Read the model definition and answer for the solid it produces. Units are mm, in the model's axes. Coordinates: 2 decimals unless noted, no trailing zeros. Loops run counter-clockwise (first coordinate to the right, second up) from the corner with the lowest first, then second, coordinate; pieces in that order, holes last.
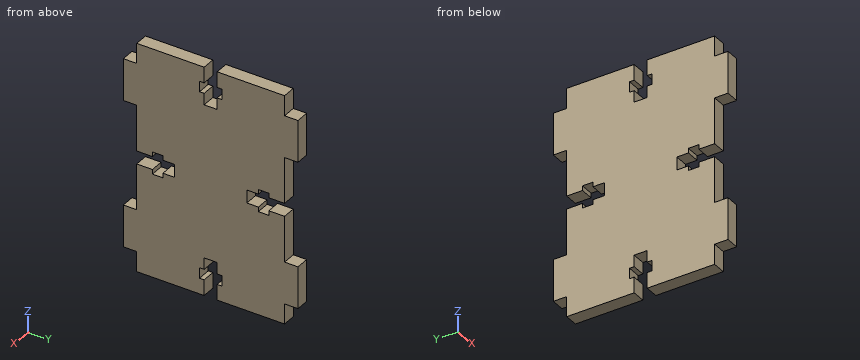
from build123d import *

# Parameters (mm, degrees)
F1_W     = 35.28
F1_H     = 54.6
F2_DEPTH = 3.2
F3_W     = 3.2
F3_H     = 10
F4_DEPTH = 3.2
F5_W     = 3.1
F5_H     = 3.75
F5_H_2   = 2.5
F5_W_2   = 1.1
F5_H_3   = 2.75
F5_W_3   = 3.75
F5_H_4   = 3.1
F5_W_4   = 2.5
F5_H_5   = 1.1
F5_W_5   = 2.75
F6_DEPTH = 3.201


with BuildPart() as f2:
    # F1 (on Right) → F2 (new body)
    with BuildSketch(Plane.YZ):
        with Locations((0, 27.3)):
            Rectangle(F1_W, F1_H)
    extrude(amount=F2_DEPTH)

    # F3 (on face) → F4 (join, through all)
    with BuildSketch(Plane.YZ.offset(3.2)):
        with Locations((-19.24, 44.8)):
            Rectangle(F3_W, F3_H)
        with Locations((-19.24, 9.8)):
            Rectangle(F3_W, F3_H)
        with Locations((19.24, 9.8)):
            Rectangle(F3_W, F3_H)
        with Locations((19.24, 44.8)):
            Rectangle(F3_W, F3_H)
    extrude(amount=-F4_DEPTH)

    # F5 (on face) → F6 (cut, through all)
    with BuildSketch(Plane.YZ.offset(3.2)):
        with Locations((0, 1.875)):
            Rectangle(F5_W, F5_H)
        with Locations((0, 5)):
            Rectangle(F5_W, F5_H_2)
        with Locations((2.1, 5)):
            Rectangle(F5_W_2, F5_H_2)
        with Locations((0, 7.625)):
            Rectangle(F5_W, F5_H_3)
        with Locations((-2.1, 5)):
            Rectangle(F5_W_2, F5_H_2)
        with Locations((-15.765, 27.3)):
            Rectangle(F5_W_3, F5_H_4)
        with Locations((-12.64, 27.3)):
            Rectangle(F5_W_4, F5_H_4)
        with Locations((-12.64, 25.2)):
            Rectangle(F5_W_4, F5_H_5)
        with Locations((-10.015, 27.3)):
            Rectangle(F5_W_5, F5_H_4)
        with Locations((-12.64, 29.4)):
            Rectangle(F5_W_4, F5_H_5)
        with Locations((12.64, 29.4)):
            Rectangle(F5_W_4, F5_H_5)
        with Locations((12.64, 27.3)):
            Rectangle(F5_W_4, F5_H_4)
        with Locations((10.015, 27.3)):
            Rectangle(F5_W_5, F5_H_4)
        with Locations((15.765, 27.3)):
            Rectangle(F5_W_3, F5_H_4)
        with Locations((12.64, 25.2)):
            Rectangle(F5_W_4, F5_H_5)
        with Locations((2.1, 49.6)):
            Rectangle(F5_W_2, F5_H_2)
        with Locations((0, 46.975)):
            Rectangle(F5_W, F5_H_3)
        with Locations((0, 49.6)):
            Rectangle(F5_W, F5_H_2)
        with Locations((0, 52.725)):
            Rectangle(F5_W, F5_H)
        with Locations((-2.1, 49.6)):
            Rectangle(F5_W_2, F5_H_2)
    extrude(amount=-F6_DEPTH, mode=Mode.SUBTRACT)


solid = f2.part
Item 1: Find the intervals of material crossed by line 1 along Z through (x, y) = (1, 2.5); line 2 along Z through (x, y) = (1.7, -9.5); line 3 along Y through (x, z) = (1.05, 3), in increasing order.
Numbers:
line 1: z = 0 to 3.75, 6.25 to 48.35, 50.85 to 54.6
line 2: z = 0 to 25.75, 28.85 to 54.6
line 3: y = -17.64 to -1.55, 1.55 to 17.64
Item 2: Given pin 1 (1.6 mm diameter, centred on x = 1, y = 0.5, fed in from +Z); pin 2 (1.6 mm diameter, centred on x = 2, z = 2, fed in from -Y); pin 3 (0.9 mm diameter, centred on x = 1.5, y = 0, fed in from -Z), each flat-ended and moving along its own axis, determine where each tip first touches the part or whether it passes through.
Numbers:
pin 1: stops at z = 45.6
pin 2: stops at y = -17.64
pin 3: stops at z = 9
Item 3: A cutting plane is placed at B-B on z = 49. Determine the outline of the cut face in (x, y), then the cut area to 3 significant figures.
Numbers:
outline: (0, -20.84) - (3.2, -20.84) - (3.2, -2.65) - (0, -2.65) - close; (0, 2.65) - (3.2, 2.65) - (3.2, 20.84) - (0, 20.84) - close
area: 116 mm2
Item 4: A cutting plane is placed at C-C on z = 22. Determine the outline of the cut face in (x, y), then the cut area to 3 significant figures.
Numbers:
outline: (0, -17.64) - (3.2, -17.64) - (3.2, 17.64) - (0, 17.64) - close
area: 113 mm2
Item 5: A cutting plane is placed at A-A on z = 8. Determine the outline of the cut face in (x, y).
Numbers:
outline: (0, -20.84) - (3.2, -20.84) - (3.2, -1.55) - (0, -1.55) - close; (0, 1.55) - (3.2, 1.55) - (3.2, 20.84) - (0, 20.84) - close
